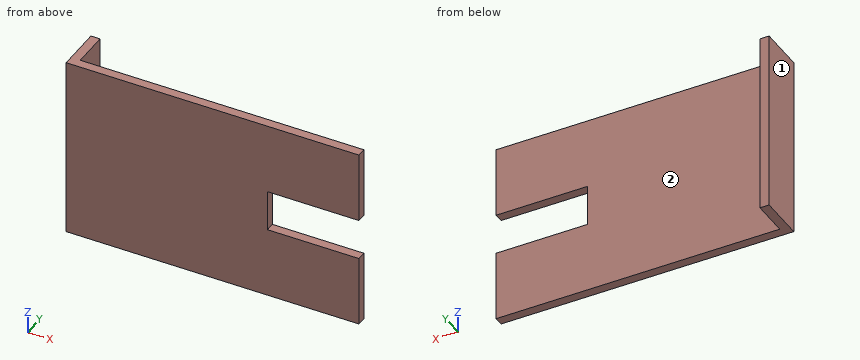
```python
from build123d import *

# Parameters (mm, degrees)
ESQUISSE1_W             = 310
ESQUISSE1_H             = 10
ESQUISSE1_W_2           = 10
ESQUISSE1_H_2           = 40
BOSS_EXTRU_1_DEPTH      = 200
ESQUISSE4_W             = 100
ESQUISSE4_H             = 45
ENL_V_MAT_EXTRU_1_DEPTH = 10


with BuildPart() as part:
    # Esquisse1 → Boss.-Extru.1 (new body)
    with BuildSketch(Plane.XY):
        with Locations((165, 5)):
            Rectangle(ESQUISSE1_W, ESQUISSE1_H)
        with Locations((5, 30)):
            Rectangle(ESQUISSE1_W_2, ESQUISSE1_H_2)
        with Locations((5, 5)):
            Rectangle(ESQUISSE1_W_2, ESQUISSE1_H)
    extrude(amount=BOSS_EXTRU_1_DEPTH)

    # Esquisse4 → Enlèv. mat.-Extru.1 (cut)
    with BuildSketch(Plane(origin=(0, 10, 0), x_dir=(1, 0, 0), z_dir=(0, 1, 0))):
        with Locations((270, -100)):
            Rectangle(ESQUISSE4_W, ESQUISSE4_H)
    extrude(amount=-ENL_V_MAT_EXTRU_1_DEPTH, mode=Mode.SUBTRACT)


solid = part.part
```
Geometry: final body of the model. Coordinates: model frame, mm. Face numbers are marked on the shaded views. A direction names the side the tool comes from. Coordinates: 2 decimals unless noted, no trailing zeros. Order: outer loops, then holes, each group sorted by start corner. A loop starts at its lowest first (then second) coordinate and runs counter-clockwise, first axis right, second up. Notation, with made-up numbers: (31.5, 17) -> (45.5, 17) arc R28 cw to (45.5, 54) -> close; hole circle Ø10 at (-16.75, -11). An arc over 180 degrees is marked (long way). Use CSV: the item, a comma, the result in double quotes.
1) Section B-B on z = 119. Output: boundary loops of the cut face in (x, y).
Findings:
outline,"(0, 0) -> (220, 0) -> (220, 10) -> (10, 10) -> (10, 50) -> (0, 50) -> close"
2) Line query: line 1 (X direction, y = 24.5, z = 76); line 2 (Z direction, x = 225, y = 4.5). Output: solid intervals per line, ascending.
Findings:
line 1,"x = 0 to 10"
line 2,"z = 0 to 77.5, 122.5 to 200"
3) Section C-C on y = 46. Output: boundary loops of the cut face in (x, z), then the cut area to 3 significant figures.
Findings:
outline,"(0, 0) -> (10, 0) -> (10, 200) -> (0, 200) -> close"
area,"2,000 mm^2"
4) Access query for the marked faces 1 and 2. Directions: +Z, -Z, +X, -X, +Y, -Y. A direction counts if a zero-diameter tool reaches every point of the face in a straight line with its end or side. Return the directions, or none.
Findings:
face 1,"+Z, -Z, -X, +Y, -Y"
face 2,"+Z, -Z, +X, +Y"
5) Pin query (flat end, axial travel): pin 1 Ø1.5 at (x, z) = (122, 123.5) entering from +Y; pin 2 Ø5 at (y, z) = (4.5, 90.5) entering from +X. Return the tip coordinate at first contact, or that it passes through.
Findings:
pin 1,"stops at y = 10"
pin 2,"stops at x = 220"
6) Section A-A on x = 240.5. Output: boundary loops of the cut face in (y, z).
Findings:
outline,"(0, 0) -> (10, 0) -> (10, 77.5) -> (0, 77.5) -> close; (0, 122.5) -> (10, 122.5) -> (10, 200) -> (0, 200) -> close"
7) Section D-D on z = 170. Output: boundary loops of the cut face in (x, y).
Findings:
outline,"(0, 0) -> (320, 0) -> (320, 10) -> (10, 10) -> (10, 50) -> (0, 50) -> close"
